The listing builds one solid part. Answer for the finished solid, in the listing's coordinates (mm). Give positions to 0.01 mm unless a question says otherwise; leave off trailing zeros. Write each loop counter-clockwise with the first axis right and the second up, starting at its lowest first coordinate (ties: lowest second). Pieces come first, ordered by that corner, then holes. Notation, with made-up numbers: (-11.75, -38) - (8.25, -38) arc R23 ccw to (8.25, -28) - close; hole circle Ø11 at (-14.75, 23.5). An arc over 180 degrees is marked (long way). Return JSON: item names as keys, results as strings.
from build123d import *

# Parameters (mm, degrees)
SKETCH9_R                               = 5
BOSS_EXTRUDE7_DEPTH                     = 7.5
SKETCH10_R                              = 4.5
BOSS_EXTRUDE8_DEPTH                     = 0.5
SKETCH11_R                              = 8
BOSS_EXTRUDE9_DEPTH                     = 40
SKETCH12_R                              = 5
BOSS_EXTRUDE10_DEPTH                    = 30
FILLET7_R                               = 1
CBORE_FOR_M6_HEX_HEAD_BOLT2_D           = 6.6
CBORE_FOR_M6_HEX_HEAD_BOLT2_DEPTH       = 10
CBORE_FOR_M6_HEX_HEAD_BOLT2_CBORE_D     = 14.547
CBORE_FOR_M6_HEX_HEAD_BOLT2_CBORE_DEPTH = 4
CBORE_FOR_M6_HEX_HEAD_BOLT2_TIP         = 1.982840043
BOSS_EXTRUDE11_START                    = 4
SKETCH27_R                              = 5
BOSS_EXTRUDE11_DEPTH                    = 4
CUT_EXTRUDE1_START                      = -5
SKETCH28_R                              = 3.3
CUT_EXTRUDE1_DEPTH                      = 5


with BuildPart() as part:
    # Sketch9 → Boss-Extrude7 (new body)
    with BuildSketch(Plane(origin=(0, 0, 0), x_dir=(1, 0, 0), z_dir=(0, 1, 0))):
        with Locations(Location((0, 0, 0), (0, 0, 270))):
            Circle(SKETCH9_R)
    extrude(amount=BOSS_EXTRUDE7_DEPTH)

    # Sketch10 → Boss-Extrude8 (add)
    with BuildSketch(Plane(origin=(0, 7.5, 0), x_dir=(1, 0, 0), z_dir=(0, 1, 0))):
        with Locations(Location((0, 0, 0), (0, 0, 270))):
            Circle(SKETCH10_R)
    extrude(amount=BOSS_EXTRUDE8_DEPTH)

    # Sketch11 → Boss-Extrude9 (add)
    with BuildSketch(Plane(origin=(0, 8, 0), x_dir=(1, 0, 0), z_dir=(0, 1, 0))):
        with Locations(Location((0, 0, 0), (0, 0, 270))):
            Circle(SKETCH11_R)
    extrude(amount=BOSS_EXTRUDE9_DEPTH)

    # Sketch12 → Boss-Extrude10 (add)
    with BuildSketch(Plane(origin=(0, 48, 0), x_dir=(1, 0, 0), z_dir=(0, 1, 0))):
        with Locations(Location((0, 0, 0), (0, 0, 270))):
            Circle(SKETCH12_R)
    extrude(amount=BOSS_EXTRUDE10_DEPTH)

    # Fillet7
    fillet7_edges = [part.edges().sort_by_distance(p)[0] for p in [
        (0, 78, -5),
    ]]
    fillet(fillet7_edges, radius=FILLET7_R)

    # CBORE for M6 Hex Head Bolt2
    with Locations(Plane(origin=(0, 0, 0), x_dir=(-1, 0, 0), z_dir=(0, -1, 0))):
        with Locations((0, 0)):
            CounterBoreHole(CBORE_FOR_M6_HEX_HEAD_BOLT2_D / 2, CBORE_FOR_M6_HEX_HEAD_BOLT2_CBORE_D / 2, CBORE_FOR_M6_HEX_HEAD_BOLT2_CBORE_DEPTH, depth=CBORE_FOR_M6_HEX_HEAD_BOLT2_DEPTH)
            with Locations((0, 0, -(CBORE_FOR_M6_HEX_HEAD_BOLT2_DEPTH + CBORE_FOR_M6_HEX_HEAD_BOLT2_TIP / 2))):  # 118° drill point
                Cone(0, CBORE_FOR_M6_HEX_HEAD_BOLT2_D / 2, CBORE_FOR_M6_HEX_HEAD_BOLT2_TIP, mode=Mode.SUBTRACT)

    # Sketch27 → Boss-Extrude11 (add)
    with BuildSketch(Plane.XZ.offset(-4).offset(BOSS_EXTRUDE11_START)):
        with Locations(Location((0, 0, 0), (0, 0, 270))):
            Circle(SKETCH27_R)
    extrude(amount=-BOSS_EXTRUDE11_DEPTH)

    # Sketch28 → Cut-Extrude1 (cut)
    with BuildSketch(Plane.XZ.offset(CUT_EXTRUDE1_START)):
        with Locations(Location((0, 0, 0), (0, 0, 270))):
            Circle(SKETCH28_R)
    extrude(amount=CUT_EXTRUDE1_DEPTH, mode=Mode.SUBTRACT)


solid = part.part
Item 1: The mould has two halves that part along Y. Classify faces 1 (the face through (0.12, 11.64, 0.56)), 2 (the face through (1.352, 7.746, 4.292)), 3 (the face through (-5.2, 48, -0.1)), 4 (the face through (-4.88, 62.3, -1.08)): +Y half, -Y half, draft (parallel to the pull), parting line (faces both ways), or undercut.
Answer below:
{"face 1": "-Y half", "face 2": "undercut", "face 3": "+Y half", "face 4": "draft"}
Item 2: A cutting plane is placed at D-D on x = -6. Determine the outline of the cut face in (y, z), then the cut area to 3 significant figures.
Answer below:
{"outline": "(8, -5.29) - (48, -5.29) - (48, 5.29) - (8, 5.29) - close", "area": "423 mm²"}
Item 3: Flat-ended cylindrical pins translate along their axes: P1, Ø1.5, axis at y = 48, z = -5, coming from the +X side; P2, Ø4, axis at y = 58, z = 0.5, coming from the -X side; P3, Ø1, axis at y = 26.5, z = -2, coming from the -X side. Find the tip coordinate at first contact, or state that the pin passes through.
Answer below:
{"P1": "stops at x = 6.78", "P2": "stops at x = -5", "P3": "stops at x = -7.86"}
Item 4: A cutting plane is placed at C-C on y = 67. Determine the outline of the cut face in (x, z), then the cut area to 3 significant figures.
Answer below:
{"outline": "circle Ø10 at (0, 0)", "area": "78.5 mm²"}
Item 5: Consider L1, parallel to X at y = 4.3, z = 0; L2, parallel to Z at x = 0.25, y = 11.5. Determine where each line is inside the solid, lowest interval first.
Answer below:
{"L1": "x = -5 to -3.3, 3.3 to 5", "L2": "z = -8 to -0.76, 0.76 to 8"}
Item 6: A cutting plane is placed at A-A on y = 22. Determine the outline of the cut face in (x, z), then the cut area to 3 significant figures.
Answer below:
{"outline": "circle Ø16 at (0, 0)", "area": "201 mm²"}
Item 7: A cutting plane is placed at B-B on x = 6.5. Determine the outline of the cut face in (y, z).
Answer below:
{"outline": "(8, -4.66) - (48, -4.66) - (48, 4.66) - (8, 4.66) - close"}
